Can you work these out from the model? Positions are in its coordinate system, mm. A direction names the side the tool comes from. Round coordinates to 2 decimals unless told otherwise and drop trailing zeros. Order: outer loops, then holes, each group sorted by start corner. A loop starts at its lowest first (then second) coordinate and runs counter-clockwise, first axis right, second up. Notation, with made-up numbers: M 48,-14 L 52,-14 A24 cw 52,14 Z; hole C 11.25,88.5 d1. An arc over 180 degrees is marked long. Answer as a JSON object with one key per item and string values. Group by question number.
from build123d import *

# Parameters (mm, degrees)
F0_W        = 67.1
F0_H        = 138.3
F0_W_2      = 21.2295074016
F0_H_2      = 8.8934414089
F1_DEPTH    = 3.55
F2_R        = 5.08
F3_T        = 2.54
F3_T3_DEPTH = 12.18


# Not quite as in the source:
# - a shell that OpenCascade refuses in one call is made with other operations: the cavity is built on its own and cut out


with BuildPart() as f1:
    # F0 (on Front) → F1 (new body, symmetric)
    with BuildSketch(Plane.XZ):
        Rectangle(F0_W, F0_H)
        with Locations((16.9262299314, 60.2459032089)):
            Rectangle(F0_W_2, F0_H_2, mode=Mode.SUBTRACT)
    extrude(amount=F1_DEPTH, both=True)

    # F2
    f2_edges = [f1.edges().sort_by_distance(p)[0] for p in [
        (33.55, 0, 69.15),
        (-33.55, 0, 69.15),
        (33.55, 0, -69.15),
        (-33.55, 0, -69.15),
    ]]
    fillet(f2_edges, radius=F2_R)

    # F3: shell of thickness 2.54, made by hand


with BuildPart() as f3_core1:
    # F3_t2: copy of F1
    add(f1.part)

    # the walls: a layer under each face that stays
    f3_faces = [f3_core1.faces().sort_by_distance(p)[0] for p in [
        (0, 0, 69.15),
        (0, 3.55, 0),
        (32.0621024484, 0, 67.6621024484),
        (-32.0621024484, 0, 67.6621024484),
        (33.55, 0, 0),
        (-33.55, 0, 0),
        (32.0621024484, 0, -67.6621024484),
        (-32.0621024484, 0, -67.6621024484),
        (0, 0, -69.15),
        (6.3114762306, 0, 60.2459032089),
        (16.9262299314, 0, 64.6926239133),
        (27.5409836322, 0, 60.2459032089),
        (16.9262299314, 0, 55.7991825044),
    ]]
    thicken(f3_faces, amount=-F3_T, mode=Mode.SUBTRACT)

    # F3_s4 → F3_t3 (cut)
    with BuildSketch(Plane.XZ.offset(-6.09)):
        Polygon((6.3368762306, 64.6672239133), (3.7714762306, 64.6926239133), (3.7714762306, 67.2326239133), (6.3114762306, 67.2326239133), align=None)
        Polygon((6.3368762306, 55.8245825044), (3.7714762306, 55.7991825044), (3.7714762306, 53.2591825044), (6.3114762306, 53.2591825044), align=None)
        Polygon((27.5155836322, 64.6672239133), (27.5409836322, 67.2326239133), (30.0809836322, 67.2326239133), (30.0809836322, 64.6926239133), align=None)
        Polygon((27.5155836322, 55.8245825044), (30.0809836322, 55.7991825044), (30.0809836322, 53.2591825044), (27.5409836322, 53.2591825044), align=None)
    extrude(amount=F3_T3_DEPTH, mode=Mode.SUBTRACT)


with BuildPart() as f1_1:
    add(f1.part)

    # what is left inside the walls is the cavity
    f3_cavity = [f3_core1.part.solids().sort_by_distance(p)[0] for p in [
        (0, -3.5246, -22.203333),
    ]]
    add(f3_cavity, mode=Mode.SUBTRACT)


solid = f1_1.part
Item 1: I need wall thicknesses on line 1 (Z direction, x = 23, y = -0.25); line 2 (X direction, y = -1.5, z = 57); line 3 (X direction, y = 0, z = 6.5). Which ranges of each line are inside material? Lowest first, please.
Item 2: Suppose I cut it at C-C, the plane z = 45. Write out the boundary of the cut face in (x, y), and give its area (3 significant figures).
Item 3: Suppose I cut it at B-B, the plane y = -2. Write out the boundary of the cut face in (x, z), and give its area (3 significant figures).
Item 4: On a 3-axis mill with a long thin cutter (end or side, diameter ignored), from which of +Z, -Z, +X, -X, +Y, -Y can I reach the whole of each face in a straight line? I mean faces 1 (the face through (-31.01, -1, -1)), 2 (the face through (32.101, -0.05, -67.622)), 3 (the face through (17, 0, 64.693)). Say none if no direction works.
Item 5: Suppose I cut it at A-A, the plane x = 17.5. Write out the boundary of the cut face in (y, z), and give its area (3 significant figures).
Item 6: I'm going to push a flat-ended pin straight in: pin 1 Ø12 at (x, z) = (0, -15) entering from -Y. Where does the tip first touch, or does it pass through?
Item 7: If we mould it in two halves opening along Z, with no side actions, what happens to faces 4 (the face through (-32.101, -0.05, -67.622)), 5 (the face through (0, -1, -66.61)), 6 (the face through (3.771, -1, 60)), 7 (the face through (0, 3.55, 1))? For each: +Z half, -Z half, draft (parallel to the pull), parting line (faces both ways), or undercut.
Item 8: Suppose I cut it at D-D, the plane x = -3. Write out the boundary of the cut face in (y, z).
Computed:
{
 "1": {"line 1": "z = -69.15 to -66.61, 53.26 to 55.8, 64.69 to 69.15", "line 2": "x = -33.55 to -31.01, 3.77 to 6.31, 27.54 to 30.08, 31.01 to 33.55", "line 3": "x = -33.55 to -31.01, 31.01 to 33.55"},
 "2": {"outline": "M -33.55,-3.55 L -31.01,-3.55 L -31.01,1.01 L 31.01,1.01 L 31.01,-3.55 L 33.55,-3.55 L 33.55,3.55 L -33.55,3.55 Z", "area": "194 mm^2"},
 "3": {"outline": "M -33.55,-64.07 A5.08 ccw -28.47,-69.15 L 28.47,-69.15 A5.08 ccw 33.55,-64.07 L 33.55,64.07 A5.08 ccw 28.47,69.15 L -28.47,69.15 A5.08 ccw -33.55,64.07 Z; hole M -31.01,-64.07 A2.54 ccw -28.47,-66.61 L 28.47,-66.61 A2.54 ccw 31.01,-64.07 L 31.01,64.07 A2.54 ccw 30.08,66.03 L 30.08,53.26 L 3.77,53.26 L 3.77,66.61 L -28.47,66.61 A2.54 ccw -31.01,64.07 Z; hole M 6.31,55.8 L 27.54,55.8 L 27.54,64.69 L 6.31,64.69 Z", "area": "1,160 mm^2"},
 "4": {"face 1": "-Y", "face 2": "-Z, +X, +Y, -Y", "face 3": "+Y, -Y"},
 "5": {"outline": "M -3.55,-69.15 L 3.55,-69.15 L 3.55,55.8 L -3.55,55.8 L -3.55,53.26 L 1.01,53.26 L 1.01,-66.61 L -3.55,-66.61 Z; M -3.55,64.69 L 3.55,64.69 L 3.55,69.15 L -3.55,69.15 Z", "area": "372 mm^2"},
 "6": {"pin 1": "stops at y = 1.01"},
 "7": {"face 4": "-Z half", "face 5": "undercut", "face 6": "undercut", "face 7": "draft"},
 "8": {"outline": "M -3.55,-69.15 L 3.55,-69.15 L 3.55,69.15 L -3.55,69.15 L -3.55,66.61 L 1.01,66.61 L 1.01,-66.61 L -3.55,-66.61 Z"}
}
